The listing builds one solid part. Answer for the finished solid, in the listing's coordinates (mm). A direction names the side the tool comes from. Round coordinates to 2 decimals unless told otherwise and drop trailing zeros. Loops run counter-clockwise (first coordinate to the right, second up) from the corner with the lowest first, then second, coordinate; pieces in that order, holes last. Notation, with made-up numbers: (67, 19.5) - (107, 19.5) arc R29 cw to (107, 44.5) - close; hole circle Ø8 at (56.25, 76). An arc over 180 degrees is marked (long way). One line per question, with ' | ' between items. Start each with the question number.
from build123d import *

# Parameters (mm, degrees)
BOSS_EXTRUDE1_DEPTH      = 30
BOSS_EXTRUDE1_TAPER      = 10
SHELL1_T                 = -5
SKETCH6_W                = 15.197518051
SKETCH6_H                = 25.772318446
BOSS_EXTRUDE4_DEPTH      = 7
SKETCH7_W                = 13.433844537
SKETCH7_H                = 5.428745395
SKETCH7_W_2              = 12.053655029
SKETCH7_H_2              = 1.978271627
CUT_EXTRUDE2_DEPTH       = 17
BOSS_EXTRUDE6_DEPTH      = 3
MIRROR9_COPY_1_DEPTH     = 3
CUT_EXTRUDE4_START       = -4
SKETCH12_R               = 2.5
CUT_EXTRUDE4_DEPTH       = 42
MIRROR11_START           = -4
MIRROR11_COPY_1_SKETCH_R = 2.5
MIRROR11_COPY_1_DEPTH    = 42


with BuildPart() as part:
    # Sketch1 → Boss-Extrude1 (new body)
    with BuildSketch(Plane.XY):
        Polygon((-100, 10.531931481), (-100, -49.468068519), (-85, -64.468068519), (35, -64.468068519), (50, -49.468068519), (50, 10.531931481), (35, 25.531931481), (-85, 25.531931481), align=None)
    extrude(amount=BOSS_EXTRUDE1_DEPTH, taper=BOSS_EXTRUDE1_TAPER)

    # Shell1
    shell1_openings = [part.faces().sort_by_distance(p)[0] for p in [
        (-25, -19.468068519, 0),
    ]]
    offset(amount=SHELL1_T, openings=shell1_openings, kind=Kind.INTERSECTION)

    # Sketch6 → Boss-Extrude4 (add)
    with BuildSketch(Plane.XY.offset(30)):
        with Locations((-66.525501272, 7.355962837)):
            Rectangle(SKETCH6_W, SKETCH6_H)
    extrude(amount=BOSS_EXTRUDE4_DEPTH)

    # Sketch7 → Cut-Extrude2 (cut)
    with BuildSketch(Plane(origin=(0, 20.24212206, 0), x_dir=(1, 0, 0), z_dir=(0, 1, 0))):
        with Locations((-66.527599538, -33.454113167)):
            Rectangle(SKETCH7_W, SKETCH7_H)
        with Locations((-66.481593222, -32.464977353)):
            Rectangle(SKETCH7_W_2, SKETCH7_H_2, mode=Mode.SUBTRACT)
    extrude(amount=-CUT_EXTRUDE2_DEPTH, mode=Mode.SUBTRACT)

    # Sketch11 → Boss-Extrude6 (add)
    with BuildSketch(Plane(origin=(0, 0, 0), x_dir=(-1, 0, 0), z_dir=(0, 0, -1))):
        Polygon((94.922866941, -47.365051148), (82.896982629, -59.390935459), (82.896982629, -69.390935459), (104.922866941, -69.390935459), (104.922866941, -47.365051148), align=None)
    boss_extrude6 = extrude(amount=BOSS_EXTRUDE6_DEPTH)

    # Mirror8: Boss-Extrude6 across plane
    add(boss_extrude6.mirror(Plane(origin=(-25, 0, 0), x_dir=(0, 0, 1), z_dir=(1, 0, 0))))

    # Mirror9: Boss-Extrude6 across plane
    add(boss_extrude6.mirror(Plane.ZX.offset(-19.468068519)))

    # Mirror9 copy 1 sketch → Mirror9 copy 1 (add)
    with BuildSketch(Plane(origin=(-50, -38.936137038, 0), x_dir=(1, 0, 0), z_dir=(0, 0, -1))):
        Polygon((94.922866941, -47.365051148), (82.896982629, -59.390935459), (82.896982629, -69.390935459), (104.922866941, -69.390935459), (104.922866941, -47.365051148), align=None)
    extrude(amount=MIRROR9_COPY_1_DEPTH)

    # Sketch12 → Cut-Extrude4 (cut)
    with BuildSketch(Plane.XY.offset(CUT_EXTRUDE4_START)):
        with Locations((-100, -64.468068519)):
            Circle(SKETCH12_R)
    cut_extrude4 = extrude(amount=CUT_EXTRUDE4_DEPTH, mode=Mode.SUBTRACT)

    # Mirror10: Cut-Extrude4 across plane
    add(cut_extrude4.mirror(Plane(origin=(-25, 0, 0), x_dir=(0, 0, 1), z_dir=(1, 0, 0))), mode=Mode.SUBTRACT)

    # Mirror11: Cut-Extrude4 across plane
    add(cut_extrude4.mirror(Plane.ZX.offset(-19.468068519)), mode=Mode.SUBTRACT)

    # Mirror11 copy 1 sketch → Mirror11 copy 1 (cut)
    with BuildSketch(Plane(origin=(-50, -38.936137038, 0), x_dir=(-1, 0, 0), z_dir=(0, 0, 1)).offset(MIRROR11_START)):
        with Locations((-100, -64.468068519)):
            Circle(MIRROR11_COPY_1_SKETCH_R)
    extrude(amount=MIRROR11_COPY_1_DEPTH, mode=Mode.SUBTRACT)


solid = part.part
(1) Each of these flat-tipped pins is pushed along its axis until it touches: P1, Ø3, axis at y = -25.5, z = 12, coming from the +X side; P2, Ø6, axis at x = 50, y = -64.47, coming from the -Z side; P3, Ø1.5, axis at y = -21.5, z = 24.5, coming from the +X side; P4, Ø4, axis at x = -98, y = -22, coming from the -Z side. Where does it stop, or does it pass through?
(2) Consider L1, parallel to Y at x = 50, z = -0.7; L2, parallel to X at y = -4.5, z = 34; L3, parallel to Z at x = -53, y = -21. Determine where each line is inside the solid, lowest interval first.
(3) Find section B-B on x = -70.5. Write down the section's boundary in (y, z), plus the area to 3 significant figures.
(4) Find section D-D on z = 7. Write down the section's boundary in (x, y), plus the area to 3 significant figures.
(5) A tool of negligible diameter and unlimited length cuts with its end or side. For faces 1 (the flat face through (-100, -47.365, -1)), 2 (the flat face through (-67.69, 20.242, 36.34)), 3 (the flat face through (-67, 12, 30.74)), from which of +Z, -Z, +X, -X, +Y, -Y can it reach the whole face along a straight path? Write none if from no direction.
(6) Find section A-A on y = -22. Write down the section's boundary in (x, z), plus the area to 3 significant figures.
(7) Determine the mould class of faces 4 (the cylindrical face through (48.66, 23.42, -1.52)), 5 (the flat face through (46, -61, 0)), 6 (the flat face through (-26, -19, 25)), 7 (the flat face through (-25.84, 22.924, 14.79)) for opening direction Y: pulls with the +Y half, pulls with the -Y half, needs draft (parallel to the pull), parting line crosses it, or undercut.
(8) Find section C-C on z = 20. Write down the section's boundary in (x, y), plus the area to 3 significant figures.
Answer below:
1) P1: x = 48.15 | P2: z = -3 | P3: x = 45.81 | P4: z = 0
2) L1: -69.39 to -66.97, -61.97 to -47.37, 8.43 to 23.03, 28.03 to 30.45 | L2: -74.12 to -58.93 | L3: 25 to 30
3) outline: (-64.47, 0) - (-59.39, 0) - (-54.98, 25) - (16.05, 25) - (20.45, 0) - (25.53, 0) - (20.24, 30) - (20.24, 30.74) - (3.24, 30.74) - (3.24, 31.48) - (20.24, 31.48) - (20.24, 33.45) - (3.24, 33.45) - (3.24, 36.17) - (20.24, 36.17) - (20.24, 37) - (-5.53, 37) - (-5.53, 30) - (-59.18, 30) - close | area: 777 mm2
4) outline: (-98.77, -48.96) - (-84.49, -63.23) - (34.49, -63.23) - (48.77, -48.96) - (48.77, 10.02) - (34.49, 24.3) - (-84.49, 24.3) - (-98.77, 10.02) - close; hole (-93.69, -46.85) - (-82.39, -58.16) - (32.39, -58.16) - (43.69, -46.85) - (43.69, 7.92) - (32.39, 19.22) - (-82.39, 19.22) - (-93.69, 7.92) - close | area: 2,130 mm2
5) face 1: -Z, +X, -X | face 2: +Z, +X, -X, +Y | face 3: +Y
6) outline: (-100, 0) - (-94.92, 0) - (-90.51, 25) - (40.51, 25) - (44.92, 0) - (50, 0) - (44.71, 30) - (-94.71, 30) - close | area: 955 mm2
7) face 4: undercut | face 5: needs draft | face 6: undercut | face 7: pulls with the +Y half
8) outline: (-96.47, -48.01) - (-83.54, -60.94) - (33.54, -60.94) - (46.47, -48.01) - (46.47, 9.07) - (33.54, 22.01) - (-83.54, 22.01) - (-96.47, 9.07) - close; hole (-91.4, -45.9) - (-81.44, -55.86) - (31.44, -55.86) - (41.4, -45.9) - (41.4, 6.97) - (31.44, 16.93) - (-81.44, 16.93) - (-91.4, 6.97) - close | area: 2,050 mm2
